from build123d import *

# Parameters (mm, degrees)
SKETCH1_W           = 68
SKETCH1_H           = 14.75
SKETCH1_W_2         = 18
BOSS_EXTRUDE1_DEPTH = 60
CUT_EXTRUDE1_REACH  = 132.065
SKETCH2_W           = 40
SKETCH2_H           = 14.75
CUT_EXTRUDE2_DEPTH  = 131.064608945
CUT_EXTRUDE3_REACH  = 132.065
SKETCH5_R           = 3.25
CUT_EXTRUDE4_REACH  = 120.778
SKETCH6_R           = 2.6
SKETCH7_R           = 2.6
CUT_EXTRUDE5_DEPTH  = 131.064608945
CUT_EXTRUDE6_REACH  = 132.065
SKETCH8_R           = 3.25
CHAMFER1_SIZE       = 1
CUT_EXTRUDE8_REACH  = 132.065
SKETCH10_R          = 3.1
SKETCH10_R_2        = 2.6
SKETCH11_W          = 18.5
SKETCH11_H          = 16
BOSS_EXTRUDE2_DEPTH = 12
SKETCH12_R          = 3.25
CUT_EXTRUDE9_DEPTH  = 119.802577834
CHAMFER2_SIZE       = 1


with BuildPart() as part:
    # Sketch1 → Boss-Extrude1 (new body)
    with BuildSketch(Plane.XY):
        Polygon((0, 0), (-29, 0), (-29, 5), (-5, 5), (-5, 52.3), (-28, 52.3), (-28, 78.05), (73, 78.05), (73, 5), (85, 5), (85, 0), (68, 0), (68, 52.3), (0, 52.3), align=None)
        with Locations((34, 64.675)):
            Rectangle(SKETCH1_W, SKETCH1_H, mode=Mode.SUBTRACT)
        with Locations((-14, 64.675)):
            Rectangle(SKETCH1_W_2, SKETCH1_H, mode=Mode.SUBTRACT)
    extrude(amount=BOSS_EXTRUDE1_DEPTH)

    # Sketch2 → Cut-Extrude1 (cut, up to next)
    with BuildSketch(Plane(origin=(0, 0, 0), x_dir=(0, 0, -1), z_dir=(1, 0, 0)), mode=Mode.PRIVATE) as cut_extrude1_sk1:
        with Locations((-30, 64.675)):
            Rectangle(SKETCH2_W, SKETCH2_H)
    cut_extrude1_tool1 = extrude(cut_extrude1_sk1.sketch, amount=-CUT_EXTRUDE1_REACH, mode=Mode.PRIVATE) & part.part
    add(cut_extrude1_tool1.solids().sort_by_distance((0, 64.675, 30))[0], mode=Mode.SUBTRACT)

    # Sketch3 → Cut-Extrude2 (cut, through all)
    with BuildSketch(Plane(origin=(0, 78.05, 0), x_dir=(1, 0, 0), z_dir=(0, 1, 0))):
        with BuildLine():
            Line((39.5, -19), (46.5, -19))
            ThreePointArc((46.5, -19), (57.5, -30), (46.5, -41))
            Line((46.5, -41), (39.5, -41))
            ThreePointArc((39.5, -41), (28.5, -30), (39.5, -19))
        make_face()
        with BuildLine():
            Line((31, -16.1), (24, -16.1))
            ThreePointArc((24, -16.1), (22.4, -14.5), (24, -12.9))
            Line((24, -12.9), (31, -12.9))
            ThreePointArc((31, -12.9), (32.6, -14.5), (31, -16.1))
        make_face()
        with BuildLine():
            Line((55, -16.1), (62, -16.1))
            ThreePointArc((62, -16.1), (63.6, -14.5), (62, -12.9))
            Line((62, -12.9), (55, -12.9))
            ThreePointArc((55, -12.9), (53.4, -14.5), (55, -16.1))
        make_face()
        with BuildLine():
            Line((31, -43.9), (24, -43.9))
            ThreePointArc((24, -43.9), (22.4, -45.5), (24, -47.1))
            Line((24, -47.1), (31, -47.1))
            ThreePointArc((31, -47.1), (32.6, -45.5), (31, -43.9))
        make_face()
        with BuildLine():
            Line((55, -43.9), (62, -43.9))
            ThreePointArc((62, -43.9), (63.6, -45.5), (62, -47.1))
            Line((62, -47.1), (55, -47.1))
            ThreePointArc((55, -47.1), (53.4, -45.5), (55, -43.9))
        make_face()
    extrude(amount=-CUT_EXTRUDE2_DEPTH, mode=Mode.SUBTRACT)

    # Sketch5 → Cut-Extrude3 (cut, up to next)
    with BuildSketch(Plane(origin=(0, 78.05, 0), x_dir=(1, 0, 0), z_dir=(0, 1, 0)), mode=Mode.PRIVATE) as cut_extrude3_sk1:
        with Locations(Location((9, -42.73, 0), (0, 0, 270))):
            Circle(SKETCH5_R)
    cut_extrude3_tool1 = extrude(cut_extrude3_sk1.sketch, amount=-CUT_EXTRUDE3_REACH, mode=Mode.PRIVATE) & part.part
    add(cut_extrude3_tool1.solids().sort_by_distance((9, 78.05, 42.73))[0], mode=Mode.SUBTRACT)

    # Sketch6 → Cut-Extrude4 (cut, up to next)
    with BuildSketch(Plane(origin=(0, 57.3, 0), x_dir=(1, 0, 0), z_dir=(0, 1, 0)), mode=Mode.PRIVATE) as cut_extrude4_sk1:
        with Locations(Location((9, -42.73, 0), (0, 0, 270))):
            Circle(SKETCH6_R)
    cut_extrude4_tool1 = extrude(cut_extrude4_sk1.sketch, amount=-CUT_EXTRUDE4_REACH, mode=Mode.PRIVATE) & part.part
    add(cut_extrude4_tool1.solids().sort_by_distance((9, 57.3, 42.73))[0], mode=Mode.SUBTRACT)

    # Sketch7 → Cut-Extrude5 (cut, through all)
    with BuildSketch(Plane(origin=(0, 78.05, 0), x_dir=(1, 0, 0), z_dir=(0, 1, 0))):
        with Locations(Location((-14, -30, 0), (0, 0, 270))):
            Circle(SKETCH7_R)
    extrude(amount=-CUT_EXTRUDE5_DEPTH, mode=Mode.SUBTRACT)

    # Sketch8 → Cut-Extrude6 (cut, up to next)
    with BuildSketch(Plane(origin=(0, 78.05, 0), x_dir=(1, 0, 0), z_dir=(0, 1, 0)), mode=Mode.PRIVATE) as cut_extrude6_sk1:
        with Locations(Location((-14, -30, 0), (0, 0, 270))):
            Circle(SKETCH8_R)
    cut_extrude6_tool1 = extrude(cut_extrude6_sk1.sketch, amount=-CUT_EXTRUDE6_REACH, mode=Mode.PRIVATE) & part.part
    add(cut_extrude6_tool1.solids().sort_by_distance((-14, 78.05, 30))[0], mode=Mode.SUBTRACT)

    # Chamfer1
    chamfer1_edges = [part.edges().sort_by_distance(p)[0] for p in [
        (9, 78.05, 39.48),
        (-14, 78.05, 26.75),
    ]]
    chamfer(chamfer1_edges, length=CHAMFER1_SIZE)

    # Sketch10 → Cut-Extrude8 (cut, up to next)
    with BuildSketch(Plane.XZ, mode=Mode.PRIVATE) as cut_extrude8_sk1:
        with Locations((-21, 45)):
            Circle(SKETCH10_R)
    cut_extrude8_tool1 = extrude(cut_extrude8_sk1.sketch, amount=-CUT_EXTRUDE8_REACH, mode=Mode.PRIVATE) & part.part
    # Sketch10 → Cut-Extrude8 (cut, up to next)
    with BuildSketch(Plane.XZ, mode=Mode.PRIVATE) as cut_extrude8_sk2:
        with Locations((-21, 15)):
            Circle(SKETCH10_R)
    cut_extrude8_tool2 = extrude(cut_extrude8_sk2.sketch, amount=-CUT_EXTRUDE8_REACH, mode=Mode.PRIVATE) & part.part
    # Sketch10 → Cut-Extrude8 (cut, up to next)
    with BuildSketch(Plane.XZ, mode=Mode.PRIVATE) as cut_extrude8_sk3:
        with Locations((79, 15)):
            Circle(SKETCH10_R_2)
    cut_extrude8_tool3 = extrude(cut_extrude8_sk3.sketch, amount=-CUT_EXTRUDE8_REACH, mode=Mode.PRIVATE) & part.part
    # Sketch10 → Cut-Extrude8 (cut, up to next)
    with BuildSketch(Plane.XZ, mode=Mode.PRIVATE) as cut_extrude8_sk4:
        with Locations((79, 45)):
            Circle(SKETCH10_R_2)
    cut_extrude8_tool4 = extrude(cut_extrude8_sk4.sketch, amount=-CUT_EXTRUDE8_REACH, mode=Mode.PRIVATE) & part.part
    add(cut_extrude8_tool1.solids().sort_by_distance((-21, 0, 45))[0], mode=Mode.SUBTRACT)
    add(cut_extrude8_tool2.solids().sort_by_distance((-21, 0, 15))[0], mode=Mode.SUBTRACT)
    add(cut_extrude8_tool3.solids().sort_by_distance((79, 0, 15))[0], mode=Mode.SUBTRACT)
    add(cut_extrude8_tool4.solids().sort_by_distance((79, 0, 45))[0], mode=Mode.SUBTRACT)

    # Sketch11 → Boss-Extrude2 (add)
    with BuildSketch(Plane.XZ.offset(-52.3)):
        with Locations((9.25, 30)):
            Rectangle(SKETCH11_W, SKETCH11_H)
    extrude(amount=BOSS_EXTRUDE2_DEPTH)

    # Sketch12 → Cut-Extrude9 (cut, through all)
    with BuildSketch(Plane(origin=(18.5, 0, 0), x_dir=(0, 0, -1), z_dir=(1, 0, 0))):
        with Locations((-29.45403853, 46.709471103)):
            Circle(SKETCH12_R)
    extrude(amount=-CUT_EXTRUDE9_DEPTH, mode=Mode.SUBTRACT)

    # Chamfer2
    chamfer2_edges = [part.edges().sort_by_distance(p)[0] for p in [
        (-5, 46.709471103, 32.70403853),
    ]]
    chamfer(chamfer2_edges, length=CHAMFER2_SIZE)


solid = part.part
Model file for the job. Use its own axes, mm. A direction names the side the tool comes from. Give positions to 0.01 mm unless a question says otherwise; leave off trailing zeros. Loops run counter-clockwise (first coordinate to the right, second up) from the corner with the lowest first, then second, coordinate; pieces in that order, holes last.
1) Flat gauge pins, fed straight in: pin 1 Ø8.5 at (x, z) = (79, 45) entering from +Y; pin 2 Ø4 at (x, z) = (9, 42.73) entering from +Y; pin 3 Ø10 at (x, z) = (54.5, 33.5) entering from -Y; pin 4 Ø12 at (y, z) = (36, 7.5) entering from -X. Where does each tip first touch, or does it go through?
2) Saw through at D-D (x = 3). Write the cut outline in (y, z), plus the area to 3 significant figures.
3) Wall check: line 1 (Z direction, x = 60, y = 72.5); line 2 (Y direction, x = -17, z = 16); line 3 (X direction, y = 55.35, z = 30). Give the ranges that are in metal, low to high.
4) Saw through at A-A (y = 24). Write the cut outline in (x, z), plus the area to 3 significant figures.
5) Saw through at C-C (z = 4). Write the cut outline in (x, y), plus the area to 3 significant figures.
6) Pull direction Z, two halves, no side cores. Call faces 4 (the flat face through (24, 54, 0)), 5 (the flat face through (22, 78.05, 30)), 6 (the flat face through (-2, 65, 50)): +Z half, -Z half, draft (parallel to the pull), parting line (faces both ways), or undercut.
7) Saw through at B-B (x = -21). Write the cut outline in (y, z), plus the area to 3 significant figures.
8) Tool access for faces 1 (the flat face through (73, 42, 30)), 2 (the cylindrical face through (-13.02, 74.58, 33.1)), 3 (the cylindrical face through (63.6, 75.1, 45.5)): list every direction of +Z, -Z, +X, -X, +Y, -Y with a clear straight run to the whole face (end or side of a thin tool).
Answer block:
1. pin 1: stops at y = 5
1. pin 2: passes through
1. pin 3: stops at y = 52.3
1. pin 4: stops at x = -5
2. outline: (40.3, 22) - (52.3, 22) - (52.3, 0) - (57.3, 0) - (57.3, 60) - (52.3, 60) - (52.3, 38) - (40.3, 38) - close; (72.05, 0) - (78.05, 0) - (78.05, 60) - (72.05, 60) - close; hole circle Ø6.5 at (46.71, 29.45)
2. area: 819 mm2
3. line 1: z = 0 to 12.9, 16.1 to 43.9, 47.1 to 60
3. line 2: y = 0 to 5, 52.3 to 57.3, 72.05 to 78.05
3. line 3: x = -28 to -16.6, -11.4 to 28.5, 57.5 to 73
4. outline: (-5, 0) - (0, 0) - (0, 60) - (-5, 60) - close; (68, 0) - (73, 0) - (73, 60) - (68, 60) - close
4. area: 600 mm2
5. outline: (-29, 0) - (0, 0) - (0, 52.3) - (68, 52.3) - (68, 0) - (85, 0) - (85, 5) - (73, 5) - (73, 78.05) - (-28, 78.05) - (-28, 52.3) - (-5, 52.3) - (-5, 5) - (-29, 5) - close; hole (-23, 57.3) - (-5, 57.3) - (-5, 72.05) - (-23, 72.05) - close; hole (0, 57.3) - (68, 57.3) - (68, 72.05) - (0, 72.05) - close
5. area: 2,040 mm2
6. face 4: -Z half
6. face 5: draft
6. face 6: undercut
7. outline: (0, 0) - (5, 0) - (5, 11.9) - (0, 11.9) - close; (0, 18.1) - (5, 18.1) - (5, 41.9) - (0, 41.9) - close; (0, 48.1) - (5, 48.1) - (5, 60) - (0, 60) - close; (52.3, 0) - (57.3, 0) - (57.3, 60) - (52.3, 60) - close; (72.05, 0) - (78.05, 0) - (78.05, 60) - (72.05, 60) - close
7. area: 898 mm2
8. face 1: +Z, -Z, +X, +Y
8. face 2: +Y
8. face 3: +Y, -Y
